Geometry check sheet. Reference: the model listing, model coordinates, mm. A direction names the side the tool comes from. Give positions to 0.01 mm unless a question says otherwise; leave off trailing zeros. Write each loop counter-clockwise with the first axis right and the second up, starting at its lowest first coordinate (ties: lowest second). Pieces come first, ordered by that corner, then holes. Notation, with made-up numbers: M 43.5,58 L 83.5,58 A30 cw 83.5,95 Z; hole C 59,68.25 d11. An arc over 180 degrees is marked long. One line per item, written item: value. Start each with the question number.
1. Cross-section at C-C on x = 56. Record the cut outline in (y, z).
2. Tool access check on faces 1 (the face through (110.99, -2.17, -9.76)), 2 (the face through (-30, -34, -10)), 3 (the face through (150, 0, 0)). Record the directions out of +Z, -Z, +X, -X, +Y, -Y that give a thin tool (end or side, any length) a straight path to the whole face; none if there is none.
3. Scan lines: line 1 (X direction, y = -38, z = 12); line 2 (X direction, y = -16.5, z = -10). Record each from-to range of solid material in increasing order.
4. Gauge pin test, flat ends, axial feed: pin 1 (1.5 mm diameter, centred on x = -97, z = 7, fed in from +Y); pin 2 (2 mm diameter, centred on x = 8, z = 31.5, fed in from +Y); pin 3 (6 mm diameter, centred on y = -9.5, z = -29.5, fed in from +X). Record the tip position at first contact, or that the pin passes through.
5. Cross-section at D-D on x = 8. Record the cut outline in (y, z), then the cut area to 3 significant figures.
from build123d import *

# Parameters (mm, degrees)
F2_R    = 5
F3_SIZE = 2
F4_R    = 5


with BuildPart() as f1:
    # F0 (on Top) → F1 (revolve)
    with BuildSketch(Plane.XY):
        Polygon((-150, 10), (-150, 0), (150, 0), (150, 10), (70, 10), (70, 30), (30, 30), (30, 50), (-30, 50), (-30, 30), (-70, 30), (-70, 10), align=None)
    revolve(axis=Axis((0, 0, 0), (1, 0, 0)))

    # F2
    f2_edges = [f1.edges().sort_by_distance(p)[0] for p in [
        (-30, -30, 0),
        (30, -30, 0),
    ]]
    fillet(f2_edges, radius=F2_R)

    # F3
    f3_edges = [f1.edges().sort_by_distance(p)[0] for p in [
        (-150, -10, 0),
        (150, -10, 0),
    ]]
    chamfer(f3_edges, length=F3_SIZE)

    # F4
    f4_edges = [f1.edges().sort_by_distance(p)[0] for p in [
        (-70, -10, 0),
        (70, -10, 0),
    ]]
    fillet(f4_edges, radius=F4_R)


solid = f1.part
Report:
1. outline: C 0,0 d60
2. face 1: +X
2. face 2: -X
2. face 3: +Z, -Z, +X, +Y, -Y
3. line 1: x = -30 to 30
3. line 2: x = -70 to 70
4. pin 1: stops at y = 7.81
4. pin 2: stops at y = 39.62
4. pin 3: stops at x = 70
5. outline: C 0,0 d100
5. area: 7,850 mm^2
